```python
from build123d import *

# Parameters (mm, degrees)
F0_W      = 2
F0_H      = 32
F0_H_2    = 3
F0_W_2    = 5
F1_DEPTH  = 25
F0_W_3    = 3
F0_W_4    = 37.5
F2_DEPTH  = 3
F3_R      = 2.6
F6_DEPTH  = 1
F7_R      = 0.99999
F10_DEPTH = 1
F11_R     = 0.99999
F12_DEPTH = 5
F13_DEPTH = 5


# Not quite as in the source:
# - a fillet or chamfer is up to 0.001 mm smaller than in the source, because OpenCascade refuses the exact size
# - a feature names something its author has since deleted; it is built from what else it names


with BuildPart() as f1:
    # F0 (on Top) → F1 (new body)
    with BuildSketch(Plane.XY):
        with Locations((-23.75, 0)):
            Rectangle(F0_W, F0_H)
        with Locations((-23.75, 17.5)):
            Rectangle(F0_W, F0_H_2)
        with Locations((-23.75, -17.5)):
            Rectangle(F0_W, F0_H_2)
        with Locations((-20.25, 17.5)):
            Rectangle(F0_W_2, F0_H_2)
        with Locations((-20.25, -17.5)):
            Rectangle(F0_W_2, F0_H_2)
    extrude(amount=F1_DEPTH)



with BuildPart() as f1b:
    # F0 (on Top) → F1, piece 2 (new body)
    with BuildSketch(Plane.XY):
        with Locations((21.25, -17.5)):
            Rectangle(F0_W_3, F0_H_2)
        with Locations((23.75, -17.5)):
            Rectangle(F0_W, F0_H_2)
        with Locations((23.75, 0)):
            Rectangle(F0_W, F0_H)
        with Locations((23.75, 17.5)):
            Rectangle(F0_W, F0_H_2)
        with Locations((21.25, 17.5)):
            Rectangle(F0_W_3, F0_H_2)
    extrude(amount=F1_DEPTH)


with BuildPart() as f1_1:
    add(f1.part)

    add(f1b.part)  # F2 merges F1b
    # F0 (on Top) → F2 (join)
    with BuildSketch(Plane.XY):
        with Locations((21.25, 0)):
            Rectangle(F0_W_3, F0_H)
        with Locations((1, 17.5)):
            Rectangle(F0_W_4, F0_H_2)
        with Locations((-20.25, 0)):
            Rectangle(F0_W_2, F0_H)
        with Locations((1, -17.5)):
            Rectangle(F0_W_4, F0_H_2)
    extrude(amount=F2_DEPTH)

    # F3
    f3_edges = [f1_1.edges().sort_by_distance(p)[0] for p in [
        (-24.75, 19, 12.5),
        (24.75, 19, 12.5),
        (24.75, -19, 12.5),
        (-24.75, -19, 12.5),
    ]]
    fillet(f3_edges, radius=F3_R)

    # F5 (on face) → F6 (join)
    with BuildSketch(Plane.YZ.offset(22.75)):
        Polygon((-11.75, 15), (-11.75, 13), (-9.25, 13), (-6.75, 13), (-6.75, 15), (-9.25, 15), align=None)
        Polygon((-2.5, 15), (-2.5, 13), (0, 13), (2.5, 13), (2.5, 15), (0, 15), align=None)
        Polygon((6.75, 15), (6.75, 13), (9.25, 13), (11.75, 13), (11.75, 15), (9.25, 15), align=None)
    extrude(amount=-F6_DEPTH)

    # F7 (radius 1 in the source; OpenCascade refuses exactly that, so slightly less here)
    f7_edges = [f1_1.edges().sort_by_distance(p)[0] for p in [
        (21.75, -9.25, 15),
        (21.75, -9.25, 13),
        (21.75, 0, 15),
        (21.75, 0, 13),
        (21.75, 9.25, 13),
        (21.75, 9.25, 15),
    ]]
    fillet(f7_edges, radius=F7_R)

    # F9 (on face) → F10 (join)
    with BuildSketch(Plane.YZ.offset(-22.75)):
        Polygon((-11.75, 15), (-11.75, 13), (-9.25, 13), (-6.75, 13), (-6.75, 15), (-9.25, 15), align=None)
        Polygon((-2.5, 15), (-2.5, 13), (0, 13), (2.5, 13), (2.5, 15), (0, 15), align=None)
        Polygon((6.75, 15), (6.75, 13), (9.25, 13), (11.75, 13), (11.75, 15), (9.25, 15), align=None)
    extrude(amount=F10_DEPTH)

    # F11 (radius 1 in the source; OpenCascade refuses exactly that, so slightly less here)
    f11_edges = [f1_1.edges().sort_by_distance(p)[0] for p in [
        (-21.75, -9.25, 15),
        (-21.75, -9.25, 13),
        (-21.75, 0, 15),
        (-21.75, 9.25, 15),
        (-21.75, 0, 13),
        (-21.75, 9.25, 13),
    ]]
    fillet(f11_edges, radius=F11_R)

    # F5 (on face) → F12 (cut)
    with BuildSketch(Plane.YZ.offset(22.75)):
        with BuildLine():
            ThreePointArc((-8.75, 15.5), (-9.6035533906, 15.8535533906), (-9.25, 15))
            ThreePointArc((-9.25, 15), (-8.8964466094, 15.1464466094), (-8.75, 15.5))
        make_face()
        with BuildLine():
            ThreePointArc((0.5, 15.5), (-0.3535533906, 15.8535533906), (0, 15))
            ThreePointArc((0, 15), (0.3535533906, 15.1464466094), (0.5, 15.5))
        make_face()
        with BuildLine():
            ThreePointArc((9.75, 15.5), (8.8964466094, 15.8535533906), (9.25, 15))
            ThreePointArc((9.25, 15), (9.6035533906, 15.1464466094), (9.75, 15.5))
        make_face()
        with BuildLine():
            ThreePointArc((9.75, 12.5), (9.6035533906, 12.8535533906), (9.25, 13))
            ThreePointArc((9.25, 13), (8.8964466094, 12.1464466094), (9.75, 12.5))
        make_face()
        with BuildLine():
            ThreePointArc((0.5, 12.5), (0.3535533906, 12.8535533906), (0, 13))
            ThreePointArc((0, 13), (-0.3535533906, 12.1464466094), (0.5, 12.5))
        make_face()
        with BuildLine():
            ThreePointArc((-8.75, 12.5), (-8.8964466094, 12.8535533906), (-9.25, 13))
            ThreePointArc((-9.25, 13), (-9.6035533906, 12.1464466094), (-8.75, 12.5))
        make_face()
    extrude(amount=F12_DEPTH, mode=Mode.SUBTRACT)

    # F9 (on face) → F13 (cut)
    with BuildSketch(Plane.YZ.offset(-22.75)):
        with BuildLine():
            ThreePointArc((-8.75, 15.5), (-9.6035533906, 15.8535533906), (-9.25, 15))
            ThreePointArc((-9.25, 15), (-8.8964466094, 15.1464466094), (-8.75, 15.5))
        make_face()
        with BuildLine():
            ThreePointArc((0.5, 15.5), (-0.3535533906, 15.8535533906), (0, 15))
            ThreePointArc((0, 15), (0.3535533906, 15.1464466094), (0.5, 15.5))
        make_face()
        with BuildLine():
            ThreePointArc((9.75, 15.5), (8.8964466094, 15.8535533906), (9.25, 15))
            ThreePointArc((9.25, 15), (9.6035533906, 15.1464466094), (9.75, 15.5))
        make_face()
        with BuildLine():
            ThreePointArc((9.75, 12.5), (9.6035533906, 12.8535533906), (9.25, 13))
            ThreePointArc((9.25, 13), (8.8964466094, 12.1464466094), (9.75, 12.5))
        make_face()
        with BuildLine():
            ThreePointArc((0.5, 12.5), (0.3535533906, 12.8535533906), (0, 13))
            ThreePointArc((0, 13), (-0.3535533906, 12.1464466094), (0.5, 12.5))
        make_face()
        with BuildLine():
            ThreePointArc((-8.75, 12.5), (-8.8964466094, 12.8535533906), (-9.25, 13))
            ThreePointArc((-9.25, 13), (-9.6035533906, 12.1464466094), (-8.75, 12.5))
        make_face()
    extrude(amount=-F13_DEPTH, mode=Mode.SUBTRACT)


solid = f1_1.part
```
Work out the finished part from the listing and answer in its coordinate system (mm). A direction names the side the tool comes from. Give positions to 0.01 mm unless a question says otherwise; leave off trailing zeros. Loops run counter-clockwise (first coordinate to the right, second up) from the corner with the lowest first, then second, coordinate; pieces in that order, holes last. Notation, with made-up numbers: (64, 89.5) -> (109, 89.5) arc R25 cw to (109, 109.5) -> close; hole circle Ø6 at (21, 83.5). An arc over 180 degrees is marked (long way). Put each result on its own line as item: value. Start each with the question number.
Item 1: Find the intervals of material crossed by L1, parallel to Z at x = -23.65, y = 9.25; L2, parallel to X at y = 0, z = 10.75; L3, parallel to X at y = 16.5, z = 15.5, in increasing order. Write a range as [from, to].
Item 2: The part is cut by section D-D (x = -19.5). Give the vertices of the cut face in (y, z).
Item 3: The part is cut by section A-A (z = 18). Give the vertices of the cut face in (x, y), then the cut area to 3 significant figures.
Item 4: Which of the six approach directions +Z, -Z, +X, -X, +Y, -Y give full straight-line access (tool end or side, diameter ignored) to faces 1 (the face through (21, 16, 14)), 2 (the face through (21, 0, 3)), 3 (the face through (-23, 0, 25)), 4 (the face through (1, -16, 1)), 5 (the face through (1, -17, 3))?
Item 5: The part is cut by section C-C (z = 1.75). Give the vertices of the cut face in (x, y).
Item 6: Each of these flat-tipped pins is pushed along its axis until it touches: P1, Ø3.5, axis at x = 8, y = -18, coming from the +Z side; P2, Ø2.5, axis at x = 21, y = 0, coming from the +Z side; P3, Ø3.5, axis at y = 18, z = 14.5, coming from the +X side. Where does it stop, or does it pass through?
Item 7: The part is cut by section B-B (x = 7.5). Give the vertices of the cut face in (y, z).
Item 8: The mould has two halves that part along X. Classify faces 6 (the face through (-24.75, 0, 10)), 7 (the face through (1, 16, 1)), 8 (the face through (0, -17, 0)): released by +X, released by -X, zero draft, split by the parting line, or undercut.
Answers below:
1. L1: [0, 12], [13, 15], [16, 25]
1. L2: [-24.75, -22.75], [22.75, 24.75]
1. L3: [-24.75, -17.75], [19.75, 24.75]
2. outline: (-19, 0) -> (19, 0) -> (19, 25) -> (16, 25) -> (16, 3) -> (-16, 3) -> (-16, 25) -> (-19, 25) -> close
3. outline: (-24.75, -16.4) arc R2.6 ccw to (-22.15, -19) -> (-17.75, -19) -> (-17.75, -16) -> (-22.75, -16) -> (-22.75, 16) -> (-17.75, 16) -> (-17.75, 19) -> (-22.15, 19) arc R2.6 ccw to (-24.75, 16.4) -> close; (19.75, -19) -> (22.15, -19) arc R2.6 ccw to (24.75, -16.4) -> (24.75, 16.4) arc R2.6 ccw to (22.15, 19) -> (19.75, 19) -> (19.75, 16) -> (22.75, 16) -> (22.75, -16) -> (19.75, -16) -> close
3. area: 194 mm2
4. face 1: +Z
4. face 2: none
4. face 3: +Z, +X, -X, +Y, -Y
4. face 4: +Z, -Z
4. face 5: +Z, +Y, -Y
5. outline: (-24.75, -16.4) arc R2.6 ccw to (-22.15, -19) -> (22.15, -19) arc R2.6 ccw to (24.75, -16.4) -> (24.75, 16.4) arc R2.6 ccw to (22.15, 19) -> (-22.15, 19) arc R2.6 ccw to (-24.75, 16.4) -> close; hole (-17.75, -16) -> (19.75, -16) -> (19.75, 16) -> (-17.75, 16) -> close
6. P1: z = 3
6. P2: z = 14.87
6. P3: x = 24.75
7. outline: (-19, 0) -> (-16, 0) -> (-16, 3) -> (-19, 3) -> close; (16, 0) -> (19, 0) -> (19, 3) -> (16, 3) -> close
8. face 6: released by -X
8. face 7: undercut
8. face 8: zero draft
